Geometry: final body of the model. Coordinates: model frame, mm. Coordinates: 2 decimals unless noted, no trailing zeros. Write each loop counter-clockwise with the first axis right and the second up, starting at its lowest first coordinate (ties: lowest second). Pieces come first, ordered by that corner, then holes. Notation, with made-up numbers: (-22.75, -15) -> (11.25, -15) arc R34 cw to (11.25, 16) -> close; hole circle Ø1 at (57.25, 6). An arc over 180 degrees is marked (long way). One line per item, written item: value.
Autodesk Inventor part; units mm, degrees
ref_plane "YZ Plane" through (0, 0, 0) normal (1, 0, 0) x (0, 1, 0)
ref_plane "XZ Plane" through (0, 0, 0) normal (0, 1, 0) x (-1, 0, 0)
ref_plane "XY Plane" through (0, 0, 0) normal (0, 0, 1) x (1, 0, 0)
sketch "Sketch1" plane through (0, 0, 0) normal (0, 1, 0) x (-1, 0, 0)
  line L0 (-1.778, 0) -> (10.668, 0)
  line L1 (0, -53.34) -> (0, 53.34)
  line L2 (8.89, -38.1) -> (0, -38.1)
  line L3 (0, -38.1) -> (0, 38.1)
  line L4 (0, 38.1) -> (8.89, 38.1)
  line L5 (8.89, 38.1) -> (8.89, -38.1)
  line L6 (8.89, -38.1) -> (0, 38.1) construction
  line L7 (0, -38.1) -> (8.89, 38.1) construction
  point P0 (0, 0)
  point P1 (4.445, 0)
  point P2 (5.08, 31.4325)
  point P3 (5.08, 0)
  point P4 (5.08, -31.4325)
  dimension "d0" = 76.2
  dimension "d1" = 8.89
  dimension "d2" = 5.08
  dimension "d3" = 31.4325
  dimension "d4" = 31.4325
extrude "Extrusion1" add sketch "Sketch1" against normal blind 3.175
fillet "Fillet1" radius 1.27 2 edges at (-8.89, -1.5875, 38.1) (-8.89, -1.5875, -38.1)
fillet "Fillet2" radius 1.27 2 edges at (0, -1.5875, 38.1) (0, -1.5875, -38.1)
hole "Hole1" at (-5.08, 0, 31.4325) at (-5.08, 0, 0) at (-5.08, 0, -31.4325) direction (0, -1, 0) diameter 2.9972 end through all
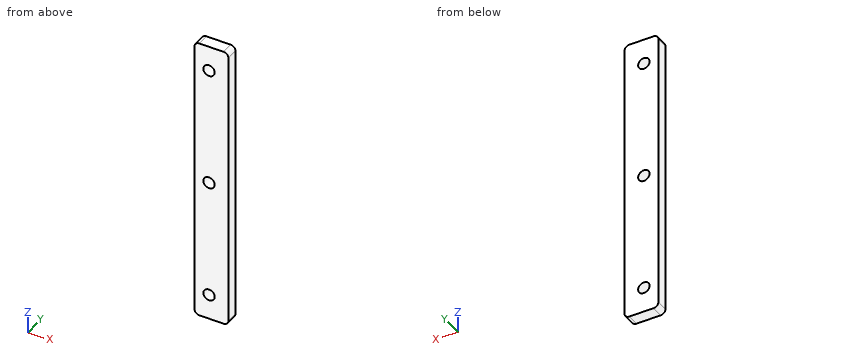
(1) Line query: line 1 (Z direction, x = -5.08, y = -0.9); line 2 (X direction, y = -1.3, z = 0); line 3 (Z direction, x = -4, y = -2.8). Output: solid intervals per line, ascending. Write a range as [from, to].
Responses:
line 1: z = [-38.1, -32.93], [-29.93, -1.5], [1.5, 29.93], [32.93, 38.1]
line 2: x = [-8.89, -6.58], [-3.58, 0]
line 3: z = [-38.1, -32.47], [-30.39, -1.04], [1.04, 30.39], [32.47, 38.1]
(2) Section A-A (y = -0.85). Return the cut outline in (x, z).
Responses:
outline: (-8.89, -36.83) arc R1.27 ccw to (-7.62, -38.1) -> (-1.27, -38.1) arc R1.27 ccw to (0, -36.83) -> (0, 36.83) arc R1.27 ccw to (-1.27, 38.1) -> (-7.62, 38.1) arc R1.27 ccw to (-8.89, 36.83) -> close; hole circle Ø3 at (-5.08, -31.43); hole circle Ø3 at (-5.08, 0); hole circle Ø3 at (-5.08, 31.43)
(3) Section B-B (z = 0). Return the cut outline in (x, y) (3 decimals), then the cut area to 3 significant figures.
Responses:
outline: (-8.89, -3.175) -> (-6.579, -3.175) -> (-6.579, 0) -> (-8.89, 0) -> close; (-3.581, -3.175) -> (0, -3.175) -> (0, 0) -> (-3.581, 0) -> close
area: 18.7 mm2
(4) Section C-C (x = -5.08). Return the cut outline in (y, z) (3 decimals), then the cut area to 3 significant figures.
Responses:
outline: (-3.175, -38.1) -> (0, -38.1) -> (0, -32.931) -> (-3.175, -32.931) -> close; (-3.175, -29.934) -> (0, -29.934) -> (0, -1.499) -> (-3.175, -1.499) -> close; (-3.175, 1.499) -> (0, 1.499) -> (0, 29.934) -> (-3.175, 29.934) -> close; (-3.175, 32.931) -> (0, 32.931) -> (0, 38.1) -> (-3.175, 38.1) -> close
area: 213 mm2
